Check sheet for the modelled part. Datum: model origin and axes. Units: mm. A direction names the side the tool comes from. Give positions to 0.01 mm unless a question says otherwise; leave off trailing zeros. Write each loop counter-clockwise with the first axis right and the second up, starting at its lowest first coordinate (ties: lowest second). Pieces come first, ordered by that corner, then holes. Notation, with made-up numbers: (62, 68) -> (87, 68) arc R14 ccw to (87, 78) -> close; hole circle Ø2 at (55, 49). An arc over 180 degrees is marked (long way). Use a Markdown table: item, result. Add a question column.
1. Gauge pin test, flat ends, axial feed: P1, Ø1.5, axis at x = -15.5, z = 1.5, coming from the +Y side; P2, Ø2.5, axis at y = -28, z = 6.5, coming from the +X side (3 decimals); P3, Ø2.5, axis at y = 26.5, z = 8, coming from the -X side (3 decimals); P4, Ø7.5, axis at x = 2.5, y = 3.5, coming from the -Z side. Record the tip position at first contact, or that the pin passes through.
2. Cross-section at D-D (y = 8.5). Enter the section's corners in (x, z) (3 decimals), then the cut area to 3 significant figures.
3. Cross-section at C-C (x = 21.5). Enter the section's corners in (y, z) (3 decimals), then the cut area to 3 significant figures.
4. Release check for a two-part mould opening along X. For faces 1 (the cylindrical face through (-8.761, -20.759, 11.976)), 2 (the cylindrical face through (21.151, -8.761, 11.976)), 3 (the cylindrical face through (3.78, 2.9, 9.37)) record: released by +X, released by -X, zero draft, split by the parting line, or undercut.
5. Set-up check for faces 4 (the cylindrical face through (8.761, -20.759, 0.724)), 5 (the cylindrical face through (-20.759, 8.761, 0.724)), 6 (the flat face through (-22, 9.525, 6)), 7 (the cylindrical face through (21.151, 8.761, 11.976)), 8 (the flat face through (0, 7.328, 3)): record each of +Z, -Z, +X, -X, +Y, -Y from which the full face is reachable in a straight line by a thin tool's end or side.
6. Cross-section at A-A (x = 0). Enter the section's corners in (y, z) (1 decimal).
7. Cross-section at B-B (z = 7.5). Enter the section's corners in (x, y) (1 decimal), then the cut area to 3 significant figures.
8. Scan lines: probe 1 along Y at (x, z) = (0, 9.25) (1 decimal); probe 2 along X at (y, z) = (24, 6) (3 decimals). Record each from-to range of solid material in increasing order. Write a range as [from, to].
from build123d import *

# Parameters (mm, degrees)
F0_W     = 19.05
F0_H     = 69.85
F1_DEPTH = 12.7
F2_W     = 69.85
F2_H     = 19.05
F3_DEPTH = 12.7
F4_R     = 2.54
F5_R     = 2.54
F7_DEPTH = 5.9436
F9_D     = 9.525


with BuildPart() as f1:
    # F0 (on Top) → F1 (new body)
    with BuildSketch(Plane.XY):
        Rectangle(F0_W, F0_H)
    extrude(amount=F1_DEPTH)

    # F2 (on Top) → F3 (join)
    with BuildSketch(Plane.XY):
        Rectangle(F2_W, F2_H)
    extrude(amount=F3_DEPTH)

    # F4
    f4_edges = [f1.edges().sort_by_distance(p)[0] for p in [
        (0, 34.925, 12.7),
        (-9.525, 22.225, 12.7),
        (-9.525, -22.225, 12.7),
        (9.525, 22.225, 12.7),
        (9.525, -22.225, 12.7),
        (-22.225, 9.525, 12.7),
        (-34.925, 0, 12.7),
        (-22.225, -9.525, 12.7),
        (0, -34.925, 12.7),
        (22.225, -9.525, 12.7),
        (34.925, 0, 12.7),
        (22.225, 9.525, 12.7),
    ]]
    fillet(f4_edges, radius=F4_R)

    # F5
    f5_edges = [f1.edges().sort_by_distance(p)[0] for p in [
        (-9.525, 22.225, 0),
        (-9.525, -22.225, 0),
        (0, -34.925, 0),
        (9.525, 22.225, 0),
        (9.525, -22.225, 0),
        (0, 34.925, 0),
        (-22.225, 9.525, 0),
        (-34.925, 0, 0),
        (-22.225, -9.525, 0),
        (22.225, -9.525, 0),
        (34.925, 0, 0),
        (22.225, 9.525, 0),
    ]]
    fillet(f5_edges, radius=F5_R)

    # F6 (on Top) → F7 (cut)
    with BuildSketch(Plane.XY):
        Polygon((-4.230765, 7.3279), (-8.46153, 0), (-4.230765, -7.3279), (4.230765, -7.3279), (8.46153, 0), (4.230765, 7.3279), align=None)
    extrude(amount=F7_DEPTH, mode=Mode.SUBTRACT)

    # F9 (through all)
    with Locations(Plane(origin=(0, 0, 0), x_dir=(1, 0, 0), z_dir=(0, 0, -1))):
        with Locations((0, 0)):
            Hole(F9_D / 2)


solid = f1.part
Worked answers:
| question | item | result |
|---|---|---|
| 1 | P1 | stops at y = 9.51 |
| 1 | P2 | stops at x = 9.525 |
| 1 | P3 | stops at x = -9.525 |
| 1 | P4 | stops at z = 0 |
| 2 | outline | (-34.925, 2.54) arc R2.54 ccw to (-33.9, 0.501) -> (-8.5, 0.501) arc R2.54 ccw to (-6.985, 0) -> (6.985, 0) arc R2.54 ccw to (8.5, 0.501) -> (33.9, 0.501) arc R2.54 ccw to (34.925, 2.54) -> (34.925, 10.16) arc R2.54 ccw to (33.9, 12.199) -> (8.5, 12.199) arc R2.54 ccw to (6.985, 12.7) -> (-6.985, 12.7) arc R2.54 ccw to (-8.5, 12.199) -> (-33.9, 12.199) arc R2.54 ccw to (-34.925, 10.16) -> close |
| 2 | area | 831 mm² |
| 3 | outline | (-9.525, 2.54) arc R2.54 ccw to (-6.985, 0) -> (6.985, 0) arc R2.54 ccw to (9.525, 2.54) -> (9.525, 10.16) arc R2.54 ccw to (6.985, 12.7) -> (-6.985, 12.7) arc R2.54 ccw to (-9.525, 10.16) -> close |
| 3 | area | 236 mm² |
| 4 | face 1 | released by -X |
| 4 | face 2 | zero draft |
| 4 | face 3 | undercut |
| 5 | face 4 | -Z, +X, -Y |
| 5 | face 5 | -Z, -X, +Y |
| 5 | face 6 | +Z, -Z, -X, +Y |
| 5 | face 7 | +Z, +X, +Y |
| 5 | face 8 | -Z |
| 6 | outline | (-34.9, 2.5) arc R2.5 ccw to (-32.4, 0) -> (-7.3, 0) -> (-7.3, 5.9) -> (-4.8, 5.9) -> (-4.8, 12.7) -> (-32.4, 12.7) arc R2.5 ccw to (-34.9, 10.2) -> close; (4.8, 5.9) -> (7.3, 5.9) -> (7.3, 0) -> (32.4, 0) arc R2.5 ccw to (34.9, 2.5) -> (34.9, 10.2) arc R2.5 ccw to (32.4, 12.7) -> (4.8, 12.7) -> close |
| 7 | outline | (-34.9, -9.5) -> (-9.5, -9.5) -> (-9.5, -34.9) -> (9.5, -34.9) -> (9.5, -9.5) -> (34.9, -9.5) -> (34.9, 9.5) -> (9.5, 9.5) -> (9.5, 34.9) -> (-9.5, 34.9) -> (-9.5, 9.5) -> (-34.9, 9.5) -> close; hole circle Ø9.5 at (0, 0) |
| 7 | area | 2,230 mm² |
| 8 | probe 1 | y = [-34.9, -4.8], [4.8, 34.9] |
| 8 | probe 2 | x = [-9.525, 9.525] |
